from build123d import *

# Parameters (mm, degrees)
SKETCH1_R           = 5
BOSS_EXTRUDE1_DEPTH = 20
SKETCH2_R           = 10
CUT_EXTRUDE1_DEPTH  = 10


with BuildPart() as part:
    # Sketch1 → Boss-Extrude1 (new body)
    with BuildSketch(Plane.XY):
        with BuildLine():
            Line((-15, 10), (-15, -10))
            ThreePointArc((-15, -10), (-8.660254038, -22.247448714), (5, -24.142135624))
            Line((5, -24.142135624), (5, -40))
            ThreePointArc((5, -40), (20, -55), (35, -40))
            Line((35, -40), (35, -15))
            Line((35, -15), (90, -15))
            ThreePointArc((90, -15), (105, 0), (90, 15))
            Line((90, 15), (35, 15))
            Line((35, 15), (35, 40))
            ThreePointArc((35, 40), (20, 55), (5, 40))
            Line((5, 40), (5, 24.142135624))
            ThreePointArc((5, 24.142135624), (-8.660254038, 22.247448714), (-15, 10))
        make_face()
        with Locations((20, 40)):
            Circle(SKETCH1_R, mode=Mode.SUBTRACT)
        with Locations((20, -40)):
            Circle(SKETCH1_R, mode=Mode.SUBTRACT)
        with Locations((90, 0)):
            Circle(SKETCH1_R, mode=Mode.SUBTRACT)
        with BuildLine():
            Line((7.5, 10), (7.5, -10))
            ThreePointArc((7.5, -10), (0, -17.5), (-7.5, -10))
            Line((-7.5, -10), (-7.5, 10))
            ThreePointArc((-7.5, 10), (0, 17.5), (7.5, 10))
        make_face(mode=Mode.SUBTRACT)
    extrude(amount=BOSS_EXTRUDE1_DEPTH)

    # Sketch2 → Cut-Extrude1 (cut)
    with BuildSketch(Plane.XY.offset(20)):
        with Locations((20, 40)):
            Circle(SKETCH2_R)
        with Locations((20, -40)):
            Circle(SKETCH2_R)
        with Locations((90, 0)):
            Circle(SKETCH2_R)
    extrude(amount=-CUT_EXTRUDE1_DEPTH, mode=Mode.SUBTRACT)


solid = part.part
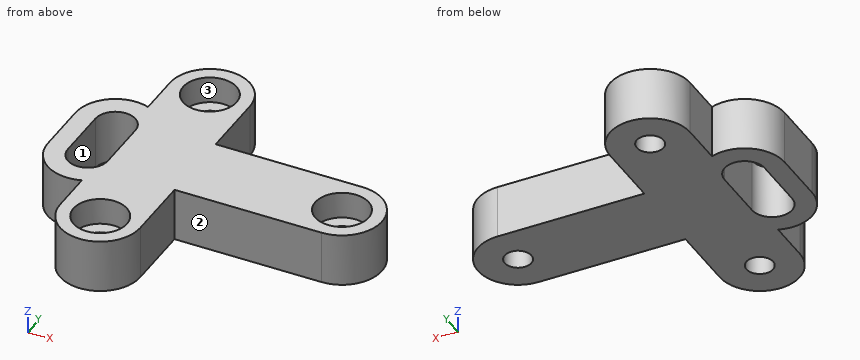
Work out the finished part from the listing and answer in its coordinate system (mm). Face numbers are marked on the shaded views. A direction names the side the tool comes from. Coordinates: 2 decimals unless noted, no trailing zeros. Loops run counter-clockwise (first coordinate to the right, second up) from the corner with the lowest first, then second, coordinate; pieces in that order, holes last. Notation, with made-up numbers: M 35,-29.5 L 73,-29.5 A16 ccw 73,-8.5 Z; hole C 26.25,40.5 d1. An arc over 180 degrees is marked long. Answer in a Markdown table with one row per item. Add a question column.
1. A tool of negligible diameter and unlimited length cuts with its end or side. For the marked faces 1, 2 and 3, from which of +Z, -Z, +X, -X, +Y, -Y can it reach the whole face along a straight path? Write none if from no direction.
2. Find section D-D, the plane x = 20. Write down the section's boundary in (y, z), then the cut area to 3 significant figures.
3. Find section A-A, the plane z = 7. Write down the section's boundary in (x, y).
4. Find section C-C, the plane y = 0. Write down the section's boundary in (x, z), then the cut area to 3 significant figures.
5. Consider L1, parallel to Y at x = 20, z = 3; L2, parallel to Y at x = 20, z = 17.5; L3, parallel to X at y = 40, z = 7.25. Determine where each line is inside the solid, lowest interval first.
6. Find section B-B, the plane x = 0. Write down the section's boundary in (y, z), then the cut area to 3 significant figures.
7. Flat-ended cylindrical pins translate along their axes: P1, Ø16, axis at x = 20, y = 40, coming from the +Z side; P2, Ø9, axis at x = 90, y = 0, coming from the +Z side; P3, Ø6, axis at x = 38.5, z = 14.5, coming from the -Y side; P4, Ø12, axis at x = 53, z = 12.5, coming from the +Y side. Find the tip coordinate at first contact, or state that the pin passes through.
Reported:
| question | item | result |
|---|---|---|
| 1 | face 1 | +Z, -Z |
| 1 | face 2 | +Z, -Z, +X, -Y |
| 1 | face 3 | +Z |
| 2 | outline | M -55,0 L -45,0 L -45,10 L -50,10 L -50,20 L -55,20 Z; M -35,0 L 35,0 L 35,10 L 30,10 L 30,20 L -30,20 L -30,10 L -35,10 Z; M 45,0 L 55,0 L 55,20 L 50,20 L 50,10 L 45,10 Z |
| 2 | area | 1,600 mm^2 |
| 3 | outline | M -15,-10 A15 ccw 5,-24.14 L 5,-40 A15 ccw 35,-40 L 35,-15 L 90,-15 A15 ccw 90,15 L 35,15 L 35,40 A15 ccw 5,40 L 5,24.14 A15 ccw -15,10 Z; hole M -7.5,-10 A7.5 ccw 7.5,-10 L 7.5,10 A7.5 ccw -7.5,10 Z; hole C 20,-40 d10; hole C 20,40 d10; hole C 90,0 d10 |
| 4 | outline | M -15,0 L -7.5,0 L -7.5,20 L -15,20 Z; M 7.5,0 L 85,0 L 85,10 L 80,10 L 80,20 L 7.5,20 Z; M 95,0 L 105,0 L 105,20 L 100,20 L 100,10 L 95,10 Z |
| 4 | area | 1,800 mm^2 |
| 5 | L1 | y = -55 to -45, -35 to 35, 45 to 55 |
| 5 | L2 | y = -55 to -50, -30 to 30, 50 to 55 |
| 5 | L3 | x = 5 to 15, 25 to 35 |
| 6 | outline | M -25,0 L -17.5,0 L -17.5,20 L -25,20 Z; M 17.5,0 L 25,0 L 25,20 L 17.5,20 Z |
| 6 | area | 300 mm^2 |
| 7 | P1 | stops at z = 10 |
| 7 | P2 | passes through |
| 7 | P3 | stops at y = -15 |
| 7 | P4 | stops at y = 15 |
